Here's the drawing with two shaded views (mm, measured from the low corner). I have some questions. Coordinates: 2 decimals unless noted, no trailing zeros. Order: outer loops, then holes, each group sorted by start corner. A loop starts at its lowest first (then second) coordinate and runs counter-clockwise, first axis right, second up. Notation, with made-up numbers: (-9.75, 23) - (6.25, 23) arc R17 ccw to (6.25, 52) - close; hole circle Ø1 at (89, -36.75). An arc over 180 degrees is marked (long way). One line per item, written item: value. Start each with the question number.
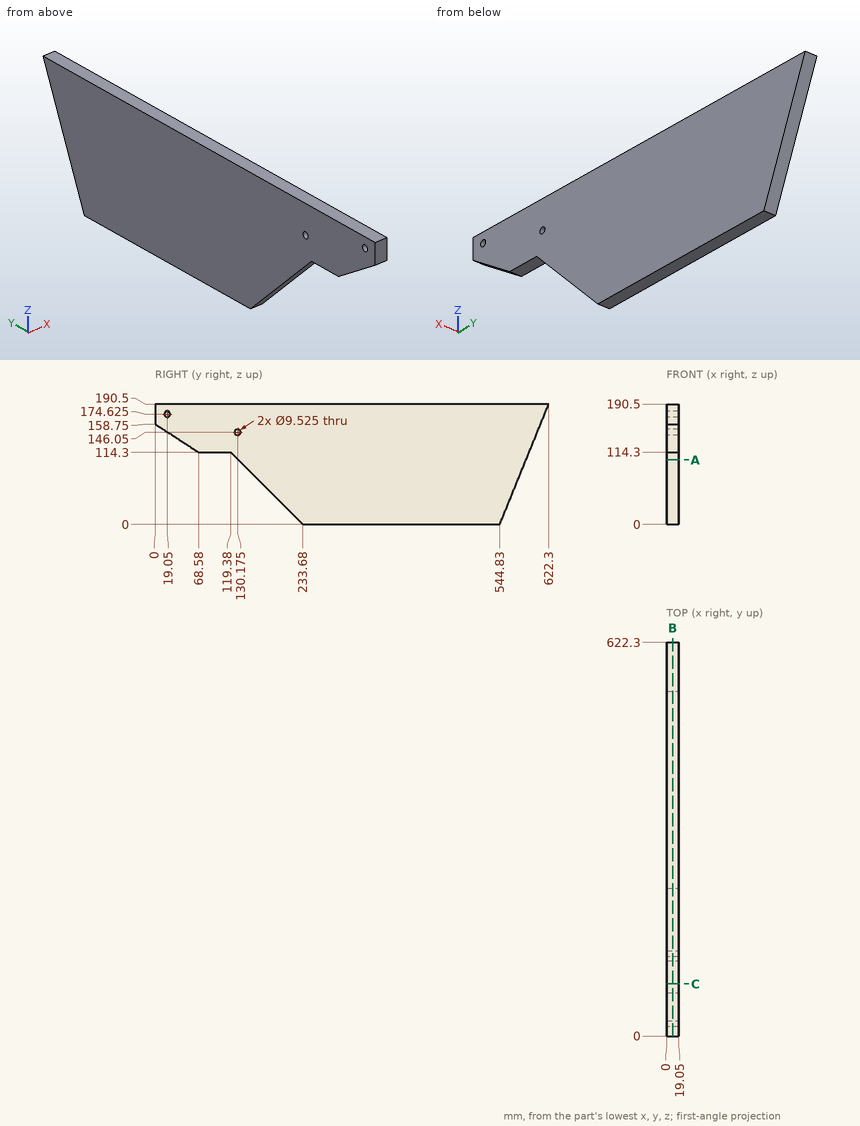
Q1. I want a section at B-B on x = 9.25. State how many separate pieces and enclosed holes the cut face has, then the cut area to 3 significant figures.
Q2. I want a section at C-C on y = 82.5. Please give me the cut outline in (x, z), then the cut area to 3 significant figures.
Q3. If I drill on L1, parallel to Y at x = 5.75, z = 146.05; L2, parallel to Z at x = 1.5, y = 85; L3, parallel to Z at x = 6.25, y = 19.05, over which ranges is the centre line in solid material (lowest first)?
Q4. I'm going to push flat-ended pins straight in: pin 1 (3 mm diameter, centred on x = 16, z = 122, fed in from -Y); pin 2 (5 mm diameter, centred on x = 11.5, z = 75.5, fed in from -Y); pin 3 (5.5 mm diameter, centred on x = 5, y = 102.5, fed in from -Z). Where does each tip first touch, or does it pass through?
Q5. I want a section at A-A on z = 102. Please give me the cut outline in (x, y), then the cut area to 3 significant figures.
Values follow:
1. separate pieces: 1
1. enclosed holes: 2
1. area: 89,300 mm^2
2. outline: (0, 114.3) - (19.05, 114.3) - (19.05, 190.5) - (0, 190.5) - close
2. area: 1,450 mm^2
3. L1: y = 19.59 to 125.41, 134.94 to 604.22
3. L2: z = 114.3 to 190.5
3. L3: z = 146.4 to 169.86, 179.39 to 190.5
4. pin 1: stops at y = 54.39
4. pin 2: stops at y = 155.68
4. pin 3: stops at z = 114.3
5. outline: (0, 131.68) - (19.05, 131.68) - (19.05, 586.31) - (0, 586.31) - close
5. area: 8,660 mm^2
